from build123d import *

# Parameters (mm, degrees)
BOSS_EXTRUDE1_DEPTH = 46
SKETCH2_R           = 4.25
CUT_EXTRUDE1_DEPTH  = 10


with BuildPart() as part:
    # Sketch1 → Boss-Extrude1 (new body)
    with BuildSketch(Plane(origin=(632.1, 0, 0), x_dir=(0, 0, -1), z_dir=(1, 0, 0))):
        with BuildLine():
            Line((277.8, -589.1), (277.8, -586.1))
            Line((277.8, -586.1), (246.077000521, -586.1))
            Line((246.077000521, -586.1), (246.077000521, -566.1))
            Line((246.077000521, -566.1), (262.077000521, -566.1))
            Line((262.077000521, -566.1), (262.077000521, -583.1))
            Line((262.077000521, -583.1), (304.643123208, -583.1))
            Line((304.643123208, -583.1), (304.643123208, -586.1))
            Line((304.643123208, -586.1), (286.8, -586.1))
            Line((286.8, -586.1), (286.8, -589.1))
            Line((286.8, -589.1), (286.8, -592.075))
            ThreePointArc((286.8, -592.075), (287.092893219, -592.782106781), (287.8, -593.075))
            Line((287.8, -593.075), (291.85, -593.075))
            Line((291.85, -593.075), (291.85, -597.842893219))
            Line((291.85, -597.842893219), (287.104675609, -602.58821761))
            ThreePointArc((287.104675609, -602.58821761), (282.3, -601.1), (277.495324391, -602.58821761))
            Line((277.495324391, -602.58821761), (272.75, -597.842893219))
            Line((272.75, -597.842893219), (272.75, -593.075))
            Line((272.75, -593.075), (276.8, -593.075))
            ThreePointArc((276.8, -593.075), (277.507106781, -592.782106781), (277.8, -592.075))
            Line((277.8, -592.075), (277.8, -589.1))
        make_face()
    extrude(amount=-BOSS_EXTRUDE1_DEPTH)

    # Sketch2 → Cut-Extrude1 (cut)
    with BuildSketch(Plane(origin=(0, -566.1, 0), x_dir=(1, 0, 0), z_dir=(0, 1, 0))):
        with Locations((608.598456538, 254.077000521)):
            Circle(SKETCH2_R)
    extrude(amount=-CUT_EXTRUDE1_DEPTH, mode=Mode.SUBTRACT)


solid = part.part
CAD build for the part. Positions are in the model's coordinates, mm. A direction names the side the tool comes from. Round coordinates to 2 decimals unless told otherwise and drop trailing zeros. Write each loop counter-clockwise with the first axis right and the second up, starting at its lowest first coordinate (ties: lowest second). Pieces come first, ordered by that corner, then holes.
(1) Slice it at D-D, the plane y = -578. Write the cut outline in (x, z).
(2) Slice it at A-A, the plane x = 615. Write the cut outline in (y, z) (3 decimals).
(3) Probe line 1 along Z through (x, y) = (600.5, -586.5); line 2 along Y through (x, z) = (611, -268); line 3 along Z through (x, y) = (601.5, -582). List the from-to ranges inside material, lowest first.
(4) Slice it at B-B, the plane z = -276. Write the cut outline in (x, y) (3 decimals).
(5) Mould opens along X. For faces 1 (the face through (609.422, -600.249, -275.156)), 2 (the face through (586.1, -585.6, -269)), 3 (the face through (612.524, -571.03, -252.449)) say: pulls with the +X half, pulls with the -X half, needs draft (parallel to the pull), parting line crosses it, or undercut.
(6) Slice it at C-C, the plane z = -253. Write the cut outline in (x, y), and give its area (3 significant figures).
(7) Drop flat-ended pins along their axis: P1, Ø3, axis at x = 624.5, z = -292, coming from the +Y side; P2, Ø6, axis at x = 617.5, z = -253.5, coming from the -Y side; P3, Ø8.5, axis at x = 602, y = -572.5, coming from the -Z side. Give the stop position or say it passes through.
(8) 3-axis set-ups, long thin cutter, end or side, ignore diameter. For faces 4 (the face through (609, -595, -272.75)), 5 (the face through (609, -593.075, -275)), 6 (the face through (609, -576.1, -254)), 7 (the face through (609, -583.1, -283)), 8 (the face through (609, -589, -286.8)): which of +Z, -Z, +X, -X, +Y, -Y reach the whole face in a straight line?
From the geometry:
1. outline: (586.1, -262.08) - (632.1, -262.08) - (632.1, -246.08) - (586.1, -246.08) - close
2. outline: (-602.588, -287.105) - (-597.843, -291.85) - (-593.075, -291.85) - (-593.075, -287.8) arc R1 cw to (-592.075, -286.8) - (-586.1, -286.8) - (-586.1, -304.643) - (-583.1, -304.643) - (-583.1, -262.077) - (-566.1, -262.077) - (-566.1, -246.077) - (-586.1, -246.077) - (-586.1, -277.8) - (-592.075, -277.8) arc R1 cw to (-593.075, -276.8) - (-593.075, -272.75) - (-597.843, -272.75) - (-602.588, -277.495) arc R8.5 cw to start
3. line 1: z = -286.8 to -277.8
3. line 2: y = -586.1 to -583.1
3. line 3: z = -262.08 to -246.08
4. outline: (586.1, -601.093) - (632.1, -601.093) - (632.1, -593.075) - (586.1, -593.075) - close; (586.1, -586.1) - (632.1, -586.1) - (632.1, -583.1) - (586.1, -583.1) - close
5. face 1: needs draft
5. face 2: pulls with the -X half
5. face 3: undercut
6. outline: (586.1, -586.1) - (632.1, -586.1) - (632.1, -566.1) - (612.71, -566.1) - (612.71, -576.1) - (604.49, -576.1) - (604.49, -566.1) - (586.1, -566.1) - close
6. area: 838 mm2
7. P1: stops at y = -583.1
7. P2: stops at y = -586.1
7. P3: stops at z = -262.08
8. face 4: +Z, +X, -X, -Y
8. face 5: +Z, +X, -X
8. face 6: +Y
8. face 7: -Z, +X, -X, +Y
8. face 8: -Z, +X, -X
